Part model, mm, in its own coordinate system. Give positions to 0.01 mm unless a question says otherwise; leave off trailing zeros. Write each loop counter-clockwise with the first axis right and the second up, starting at its lowest first coordinate (ties: lowest second). Pieces come first, ordered by that corner, then holes.
```python
from build123d import *

# Parameters (mm, degrees)
BOSS_EXTRUDE1_DEPTH    = 3.175
SKETCH2_W              = 20
SKETCH2_H              = 40
CUT_EXTRUDE1_DEPTH     = 130.299664056
M1_6_CLEARANCE_HOLE1_D = 1.7


with BuildPart() as part:
    # Sketch1 → Boss-Extrude1 (new body)
    with BuildSketch(Plane(origin=(0, 0, 0), x_dir=(1, 0, 0), z_dir=(0, 1, 0))):
        Polygon((-22.5, 0), (-22.5, 26), (22.5, 26), (22.5, 0), (28.85, 0), (28.85, -100), (22.5, -100), (22.5, -126), (-22.5, -126), (-22.5, -100), align=None)
    extrude(amount=BOSS_EXTRUDE1_DEPTH)

    # Sketch2 → Cut-Extrude1 (cut, through all)
    with BuildSketch(Plane(origin=(0, 3.175, 0), x_dir=(1, 0, 0), z_dir=(0, 1, 0))):
        with Locations((0, -4.35)):
            Rectangle(SKETCH2_W, SKETCH2_H)
    extrude(amount=-CUT_EXTRUDE1_DEPTH, mode=Mode.SUBTRACT)

    # M1.6 Clearance Hole1 (through all)
    with Locations(Plane(origin=(0, 3.175, 0), x_dir=(1, 0, 0), z_dir=(0, 1, 0))):
        with Locations((0, -28.85), (0, 20.15)):
            Hole(M1_6_CLEARANCE_HOLE1_D / 2)


solid = part.part
```
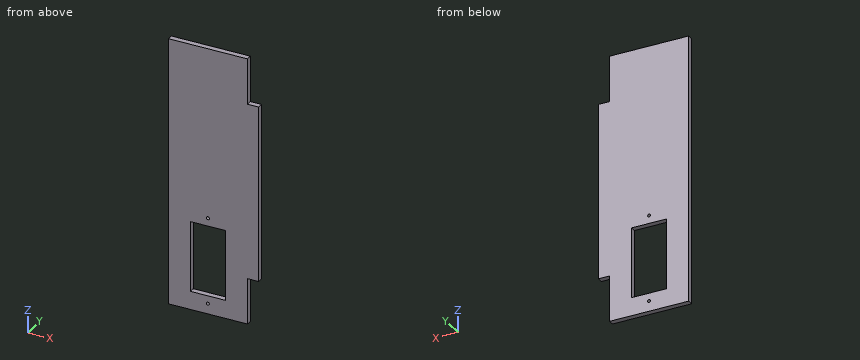
1) Wall check: L1, parallel to Z at x = 0, y = 0.85; L2, parallel to X at y = 1.5, z = 28.85; L3, parallel to Z at x = 9.5, y = 1.8. Give the ranges that are in metal, low to high.
Answers follow:
L1: z = -26 to -21, -19.3 to -15.65, 24.35 to 28, 29.7 to 126
L2: x = -22.5 to -0.85, 0.85 to 28.85
L3: z = -26 to -15.65, 24.35 to 126
2) Saw through at C-C, the plane y = 2.5. Write the cut outline in (x, z).
Answers follow:
outline: (-22.5, -26) - (22.5, -26) - (22.5, 0) - (28.85, 0) - (28.85, 100) - (22.5, 100) - (22.5, 126) - (-22.5, 126) - close; hole (-10, -15.65) - (10, -15.65) - (10, 24.35) - (-10, 24.35) - close; hole circle Ø1.7 at (0, -20.15); hole circle Ø1.7 at (0, 28.85)
3) Pin check, flat tips, straight feed: pin 1 Ø1 at (x, y) = (27, 2) entering from -Z; pin 2 Ø1.6 at (y, z) = (2.5, 110.5) entering from +X. Stop position of each tip, or through.
Answers follow:
pin 1: stops at z = 0
pin 2: stops at x = 22.5
4) Saw through at A-A, the plane x = -7.5. Write the cut outline in (y, z) (3 decimals).
Answers follow:
outline: (0, -26) - (3.175, -26) - (3.175, -15.65) - (0, -15.65) - close; (0, 24.35) - (3.175, 24.35) - (3.175, 126) - (0, 126) - close
5) Saw through at B-B, the plane z = -3. Write the cut outline in (x, y) (3 decimals).
Answers follow:
outline: (-22.5, 0) - (-10, 0) - (-10, 3.175) - (-22.5, 3.175) - close; (10, 0) - (22.5, 0) - (22.5, 3.175) - (10, 3.175) - close
6) Saw through at D-D, the plane x = 24.5. Write the cut outline in (y, z) (3 decimals), then the cut area to 4 significant figures.
Answers follow:
outline: (0, 0) - (3.175, 0) - (3.175, 100) - (0, 100) - close
area: 317.5 mm2
